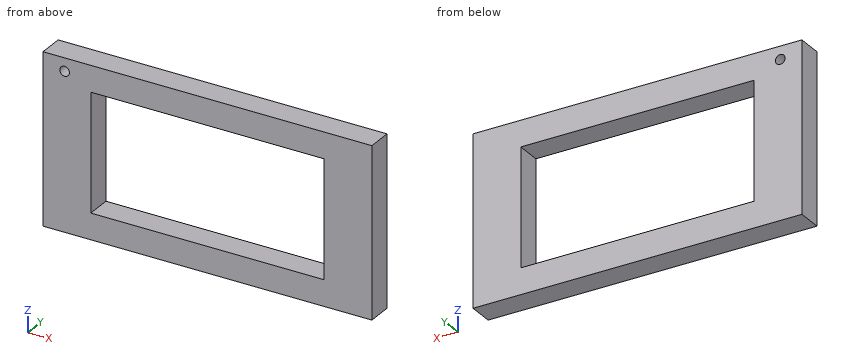
from build123d import *

# Parameters (mm, degrees)
SKETCH_W        = 34.16
SKETCH_H        = 17.6
PAD_DEPTH       = 2.6
SKETCH002_W     = 24.23
SKETCH002_H     = 12.2
POCKET_DEPTH    = 2.6
SKETCH003_R     = 0.5
SKETCH003_W     = 2.01
SKETCH003_H     = 3.5
POCKET001_DEPTH = 5


with BuildPart() as part:
    # Sketch → Pad (new body)
    with BuildSketch(Plane.XZ):
        with Locations((17.08, 8.8)):
            Rectangle(SKETCH_W, SKETCH_H)
    extrude(amount=PAD_DEPTH)

    # Sketch002 (on Face6 of Pad) → Pocket (cut)
    with BuildSketch(Plane.XZ.offset(2.6)):
        with Locations((17.08, 8.8)):
            Rectangle(SKETCH002_W, SKETCH002_H)
    extrude(amount=-POCKET_DEPTH, mode=Mode.SUBTRACT)

    # Sketch003 (on Face4 of Pocket) → Pocket001 (cut)
    with BuildSketch(Plane(origin=(0, 0, 0), x_dir=(1, 0, 0), z_dir=(0, 1, 0))):
        with Locations((2.245, -16.25)):
            Circle(SKETCH003_R)
        with Locations((27.953742, -8.544061)):
            Rectangle(SKETCH003_W, SKETCH003_H)
    extrude(amount=-POCKET001_DEPTH, mode=Mode.SUBTRACT)


solid = part.part
Geometry: final body of the model. Coordinates: model frame, mm. Coordinates: 2 decimals unless noted, no trailing zeros. Order: outer loops, then holes, each group sorted by start corner. A loop starts at its lowest first (then second) coordinate and runs counter-clockwise, first axis right, second up.
1) Section B-B (y = -0.5). Return loops of the section in (x, z) (3 decimals).
Result sheet:
outline: (0, 0) - (34.16, 0) - (34.16, 17.6) - (0, 17.6) - close; hole circle Ø1 at (2.245, 16.25); hole (4.965, 2.7) - (29.195, 2.7) - (29.195, 14.9) - (4.965, 14.9) - close
2) First-contact query: P1, Ø1.3, axis at y = -1, z = 6, coming from the -X side. Flat tip, straight axial feed; report the tip coordinate or a pass-through.
Result sheet:
P1: stops at x = 0
3) Section A-A (z = 11.75). Return loops of the section in (x, y) (3 decimals).
Result sheet:
outline: (0, -2.6) - (4.965, -2.6) - (4.965, 0) - (0, 0) - close; (29.195, -2.6) - (34.16, -2.6) - (34.16, 0) - (29.195, 0) - close
4) Ray query, probe 1 along Z at (x, y) = (8, -0.15); probe 2 along X at (y, z) = (-1.7, 4.75) (3 decimals); probe 3 along X at (y, z) = (-1.2, 16.25) (3 decimals). Return the intervals inside material, ascending.
Result sheet:
probe 1: z = 0 to 2.7, 14.9 to 17.6
probe 2: x = 0 to 4.965, 29.195 to 34.16
probe 3: x = 0 to 1.745, 2.745 to 34.16
5) Section C-C (x = 8). Return loops of the section in (y, z).
Result sheet:
outline: (-2.6, 0) - (0, 0) - (0, 2.7) - (-2.6, 2.7) - close; (-2.6, 14.9) - (0, 14.9) - (0, 17.6) - (-2.6, 17.6) - close
